Part print with two shaded views. Sizes in mm from the minimum x, y, z corner. Give positions to 0.01 mm unless a question says otherwise; leave off trailing zeros. Write each loop counter-clockwise with the first axis right and the second up, starting at its lowest first coordinate (ties: lowest second). Pieces come first, ordered by that corner, then holes. Notation, with made-up numbers: (13.5, 35.5) - (24.5, 35.5) arc R18 cw to (24.5, 62.5) - close; hole circle Ø8 at (2, 71.25). An arc over 180 degrees is marked (long way). Answer as a JSON object with one key per item and string values.
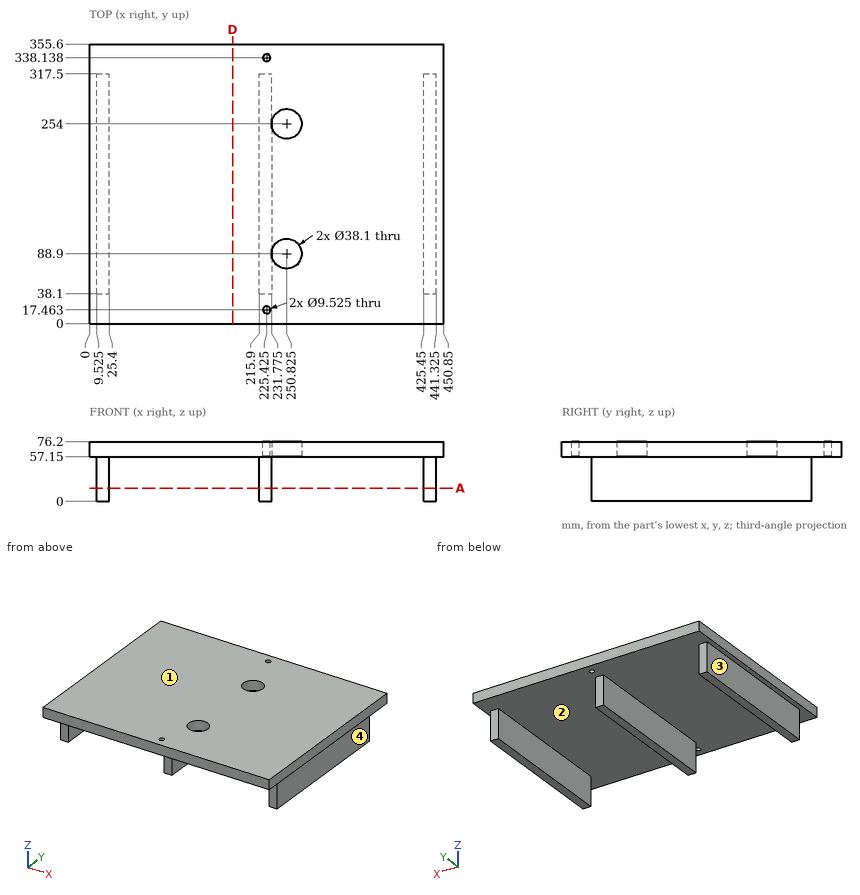
(1) Pull direction X, two halves, no side cores. Call the marked faces 1, 2, 3 and 4: pulls with the +X half, pulls with the -X half, needs draft (parallel to the pull), parting line crosses it, or undercut.
Answer key:
{"face 1": "needs draft", "face 2": "undercut", "face 3": "pulls with the -X half", "face 4": "pulls with the +X half"}
(2) Saw through at D-D, the plane x = 182. Give the cut face in (y, z), and give its area (3 significant figures).
Answer key:
{"outline": "(0, 57.15) - (355.6, 57.15) - (355.6, 76.2) - (0, 76.2) - close", "area": "6,770 mm²"}
(3) Probe L1, parallel to Z at x = 34, y = 194.5. List the from-to ranges inside material, lowest first. Write a range as [from, to].
Answer key:
{"L1": "z = [57.15, 76.2]"}
(4) Flat gauge pins, fed straight in: P1, Ø15, axis at x = 225.42, y = 338.14, coming from the -Z side; P2, Ø8, axis at y = 180, z = 29, coming from the +X side (1 decimal); P3, Ø17.5, axis at x = 437, z = 34, coming from the +Y side. Where does each tip first touch, or does it go through?
Answer key:
{"P1": "stops at z = 57.15", "P2": "stops at x = 441.3", "P3": "stops at y = 317.5"}
(5) Saw through at A-A, the plane z = 17. State how many separate pieces and enclosed holes the cut face has, and give its area (3 significant figures).
Answer key:
{"separate pieces": "3", "enclosed holes": "0", "area": "13,300 mm²"}
